from build123d import *

# Parameters (mm, degrees)
BOSS_EXTRUDE1_DEPTH = 6.35
BOSS_EXTRUDE3_DEPTH = 25.4
CUT_EXTRUDE2_DEPTH  = 6.35


with BuildPart() as part:
    # Sketch1 → Boss-Extrude1 (new body)
    with BuildSketch(Plane(origin=(0, 0, 0), x_dir=(1, 0, 0), z_dir=(0, 1, 0))):
        with BuildLine():
            Line((0.000313665, 57.24265935), (199.999794406, 33.65314008))
            ThreePointArc((199.999794406, 33.65314008), (231.692215245, 1.96024222), (199.999317386, -29.732178619))
            Line((199.999317386, -29.732178619), (-0.001522287, -57.242659331))
            ThreePointArc((-0.001522287, -57.242659331), (-57.242659343, 0.000917976), (0.000313665, 57.24265935))
        make_face()
    extrude(amount=BOSS_EXTRUDE1_DEPTH)

    # Sketch5 → Boss-Extrude3 (add)
    with BuildSketch(Plane(origin=(0, 6.35, 0), x_dir=(1, 0, 0), z_dir=(0, 1, 0))):
        with BuildLine():
            Line((0.000313665, 57.24265935), (199.999794406, 33.65314008))
            ThreePointArc((199.999794406, 33.65314008), (231.692215246, 1.960361475), (199.999555896, -29.73217862))
            Line((199.999555896, -29.73217862), (-0.001522287, -57.242659331))
            ThreePointArc((-0.001522287, -57.242659331), (-57.242659343, 0.000917976), (0.000313665, 57.24265935))
        make_face()
        with BuildLine():
            Line((-0.10621345, 44.55), (199.893342446, 20.95048073))
            ThreePointArc((199.893342446, 20.95048073), (218.989852926, 1.96048073), (199.893342446, -17.02951927))
            Line((199.893342446, -17.02951927), (-0.10621345, -44.55))
            ThreePointArc((-0.10621345, -44.55), (-44.550126614, 0), (-0.10621345, 44.55))
        make_face(mode=Mode.SUBTRACT)
    extrude(amount=BOSS_EXTRUDE3_DEPTH)

    # Sketch6 → Cut-Extrude2 (cut)
    with BuildSketch(Plane(origin=(0, 31.75, 0), x_dir=(1, 0, 0), z_dir=(0, 1, 0))):
        with BuildLine():
            Line((0, 50.9), (199.999555896, 27.30048073))
            ThreePointArc((199.999555896, 27.30048073), (225.339555896, 1.96048073), (199.999555896, -23.37951927))
            Line((199.999555896, -23.37951927), (0, -50.9))
            ThreePointArc((0, -50.9), (-50.9, 0), (0, 50.9))
        make_face()
    extrude(amount=-CUT_EXTRUDE2_DEPTH, mode=Mode.SUBTRACT)


solid = part.part
Could you check a few things on this model? Use its own coordinates, in mm. A direction names the side the tool comes from. Give positions to 0.01 mm unless a question says otherwise; leave off trailing zeros. Loops run counter-clockwise (first coordinate to the right, second up) from the corner with the lowest first, then second, coordinate; pieces in that order, holes last. Notation, with made-up numbers: (21.25, -30.75) -> (34.25, -30.75) arc R5 cw to (34.25, -25.75) -> close; hole circle Ø9 at (-19, -29.75). An arc over 180 degrees is marked (long way). Return JSON: item names as keys, results as strings.
Item 1: I need wall thicknesses on L1, parallel to Y at x = 79, z = 16; L2, parallel to Y at x = 189.5, z = -23; L3, parallel to Z at x = 139.5, y = 10. Which ranges of each line are inside material? Lowest first, please. Write a range as from..to.
Geometry results:
{"L1": "y = 0..6.35", "L2": "y = 0..25.4", "L3": "z = -40.79..-28.08, 25.34..38.05"}
Item 2: Which directions (+Z, -Z, +X, -X, +Y, -Y) give clear straight access to the entire face, cutting with the end or side of a thin tool? Please do faces 1 (the flat face through (98.6, 28.619, -39.265)), 2 (the flat face through (101.399, 3.131, 43.295)).
Geometry results:
{"face 1": "+Y", "face 2": "+Z, +X, +Y, -Y"}
Item 3: I'm going to push flat-ended pins straight in: pin 1 (3 mm diameter, centred on x = 3, y = 9, fed in from +Z); pin 2 (12 mm diameter, centred on x = 47.5, y = 20, fed in from +Z); pin 3 (3 mm diameter, centred on y = 4, z = -6.5, fed in from -X). Where does each tip first touch, or does it pass through?
Geometry results:
{"pin 1": "stops at z = 57.04", "pin 2": "stops at z = 51.53", "pin 3": "stops at x = -57.02"}
Item 4: If we section it at A-A on y = 9: List the corners of the cut face in (x, z) for me, plus the area to 3 significant figures.
Geometry results:
{"outline": "(0, -57.24) -> (200, -33.65) arc R31.69 ccw to (200, 29.73) -> (0, 57.24) arc R57.24 ccw to start; hole (-0.11, -44.55) -> (199.89, -20.95) arc R18.99 ccw (long way) to (199.89, 17.03) -> (-0.11, 44.55) arc R44.55 ccw to start", "area": "8,130 mm²"}
Item 5: If we section it at C-C on z = -41: List the corners of the cut face in (x, y) for me, plus the area to 3 significant figures.
Geometry results:
{"outline": "(-39.95, 0) -> (137.71, 0) -> (137.71, 31.75) -> (83.9, 31.75) -> (83.9, 25.4) -> (29.98, 25.4) -> (29.98, 6.35) -> (-17.43, 6.35) -> (-17.43, 25.4) -> (-30.16, 25.4) -> (-30.16, 31.75) -> (-39.95, 31.75) -> close", "area": "4,010 mm²"}
Item 6: We'd pull the mould along Z, two halves only. Please class faces 3 (the flat face through (98.494, 15.742, -32.915)), 4 (the flat face through (101.399, 18.872, 43.295)), 5 (the cylindrical face through (225.333, 28.619, -2.518)), 6 (the flat face through (98.6, 15.653, -45.613)): +Z half, -Z half, draft (parallel to the pull), parting line (faces both ways), or undercut.
Geometry results:
{"face 3": "undercut", "face 4": "+Z half", "face 5": "undercut", "face 6": "-Z half"}
